Geometry check sheet. Reference: the model listing, model coordinates, mm. A direction names the side the tool comes from. Give positions to 0.01 mm unless a question says otherwise; leave off trailing zeros. Write item = value, one per line. Start each with the question number.
1. Depth check by flat-ended pin: P1, Ø1.3, axis at x = 50.5, z = -3.5, coming from the +Y side; P2, Ø0.6, axis at x = 52.5, z = -1.5, coming from the +Y side; P3, Ø10, axis at y = 2.5, z = 2, coming from the -X side; P4, Ø6, axis at y = 0, z = -9, coming from the +X side. Enter the tip coordinate at first touch or a pass-through.
2. Thickness scan on line 1 along X through (y, z) = (17.35, -4.75); line 2 along X through (y, z) = (8.5, 0); line 3 along Z through (x, y) = (50.5, 17.35) (3 decimals). Record the ranges inside material, lowest first.
3. Mould release check, pull along Y, two halves, no side actions. Record for faces 4 (the cylindrical face through (-52.247, 11.922, 5.734)), 5 (the cylindrical face through (-52.246, 11.984, -10.672)), 6 (the cylindrical face through (51.359, 0.231, 8.797)), 7 (the flat face through (48, 17.25, -5)): pulls with the +Y half, pulls with the -Y half, needs draft (parallel to the pull), parting line crosses it, or undercut.
4. Set-up check for faces 1 (the flat face through (48, 17.25, 0)), 2 (the flat face through (52, 0, -2)), 3 (the cylindrical face through (-52.246, -11.922, -10.734)): record each of +Z, -Z, +X, -X, +Y, -Y from which the full face is reachable in a straight line by a thin tool's end or side.
```python
from build123d import *

# Parameters (mm, degrees)
SKETCH1_W           = 105
SKETCH1_H           = 35
BOSS_EXTRUDE1_DEPTH = 25
CUT_EXTRUDE1_DEPTH  = 0.5
CUT_EXTRUDE2_START  = -0.5
CUT_EXTRUDE2_DEPTH  = 0.5
FILLET1_R           = 4
FILLET2_R           = 1
SKETCH5_R           = 2
CUT_EXTRUDE3_DEPTH  = 0.25
CUT_EXTRUDE4_DEPTH  = 0.25


with BuildPart() as part:
    # Sketch1 → Boss-Extrude1 (new body)
    with BuildSketch(Plane(origin=(0, 0, -15), x_dir=(-1, 0, 0), z_dir=(0, 0, -1))):
        Rectangle(SKETCH1_W, SKETCH1_H)
    extrude(amount=-BOSS_EXTRUDE1_DEPTH)

    # Sketch2 → Cut-Extrude1 (cut)
    with BuildSketch(Plane(origin=(52.5, 0, 0), x_dir=(0, 0, -1), z_dir=(1, 0, 0))):
        with BuildLine():
            Line((-6.875, 9.125), (-6.875, -9.125))
            ThreePointArc((-6.875, -9.125), (-5.703427125, -11.953427125), (-2.875, -13.125))
            Line((-2.875, -13.125), (7.875, -13.125))
            ThreePointArc((7.875, -13.125), (10.703427125, -11.953427125), (11.875, -9.125))
            Line((11.875, -9.125), (11.875, 9.125))
            ThreePointArc((11.875, 9.125), (10.703427125, 11.953427125), (7.875, 13.125))
            Line((7.875, 13.125), (-2.875, 13.125))
            ThreePointArc((-2.875, 13.125), (-5.703427125, 11.953427125), (-6.875, 9.125))
        make_face()
    extrude(amount=-CUT_EXTRUDE1_DEPTH, mode=Mode.SUBTRACT)

    # Sketch3 → Cut-Extrude2 (cut)
    with BuildSketch(Plane.ZY.offset(52.5).offset(CUT_EXTRUDE2_START)):
        with BuildLine():
            Line((2.875, 13.125), (-7.875, 13.125))
            ThreePointArc((-7.875, 13.125), (-10.703427125, 11.953427125), (-11.875, 9.125))
            Line((-11.875, 9.125), (-11.875, -9.125))
            ThreePointArc((-11.875, -9.125), (-10.703427125, -11.953427125), (-7.875, -13.125))
            Line((-7.875, -13.125), (2.875, -13.125))
            ThreePointArc((2.875, -13.125), (5.703427125, -11.953427125), (6.875, -9.125))
            Line((6.875, -9.125), (6.875, 9.125))
            ThreePointArc((6.875, 9.125), (5.703427125, 11.953427125), (2.875, 13.125))
        make_face()
    extrude(amount=CUT_EXTRUDE2_DEPTH, mode=Mode.SUBTRACT)

    # Fillet1
    # the kernel refuses this fillet: 4 mm, written as the material it takes off along each edge
    with BuildSketch(Plane(origin=(-52.5, -27.5, -15), x_dir=(0, 0, 1), z_dir=(0, 1, 0)), Plane(origin=(52.5, 27.5, -15), x_dir=(0, 0, 1), z_dir=(0, -1, 0))) as fillet1_piece_1:
        with BuildLine():
            CenterArc((FILLET1_R, FILLET1_R), FILLET1_R, 180, 90)
            Line((0, FILLET1_R), (0, 0))
            Line((0, 0), (FILLET1_R, 0))
        make_face()
    extrude(amount=55, mode=Mode.SUBTRACT)
    with BuildSketch(Plane(origin=(-52.5, -27.5, 10), x_dir=(0, 0, -1), z_dir=(0, 1, 0)), Plane(origin=(52.5, 27.5, 10), x_dir=(0, 0, -1), z_dir=(0, -1, 0))) as fillet1_piece_2:
        with BuildLine():
            CenterArc((FILLET1_R, -FILLET1_R), FILLET1_R, 90, 90)
            Line((0, -FILLET1_R), (0, 0))
            Line((0, 0), (FILLET1_R, 0))
        make_face()
    extrude(amount=55, mode=Mode.SUBTRACT)

    # Fillet2
    fillet2_edges = [part.edges().sort_by_distance(p)[0] for p in [
        (0, -17.5, -15),
        (0, 17.5, -15),
        (-52.5, 17.5, -2.5),
        (0, 17.5, 10),
        (52.5, 17.5, -2.5),
        (51.328427125, 17.5, 8.828427125),
        (51.328427125, 17.5, -13.828427125),
        (-51.328427125, 17.5, 8.828427125),
        (-51.328427125, 17.5, -13.828427125),
        (-52.5, -17.5, -2.5),
        (52.5, -17.5, -2.5),
        (0, -17.5, 10),
        (51.328427125, -17.5, 8.828427125),
        (51.328427125, -17.5, -13.828427125),
        (-51.328427125, -17.5, 8.828427125),
        (-51.328427125, -17.5, -13.828427125),
    ]]
    fillet(fillet2_edges, radius=FILLET2_R)

    # Sketch5 → Cut-Extrude3 (cut)
    with BuildSketch(Plane(origin=(0, 17.5, 0), x_dir=(1, 0, 0), z_dir=(0, 1, 0))):
        with Locations(Location((47.5, 0.25, 0), (0, 0, 270))):
            Circle(SKETCH5_R)
        with Locations(Location((47.5, 4.75, 0), (0, 0, 270))):
            Circle(SKETCH5_R)
    extrude(amount=-CUT_EXTRUDE3_DEPTH, mode=Mode.SUBTRACT)

    # Sketch6 → Cut-Extrude4 (cut)
    with BuildSketch(Plane(origin=(0, 17.5, 0), x_dir=(1, 0, 0), z_dir=(0, 1, 0))):
        with BuildLine():
            ThreePointArc((50.671391365, 3.65), (50.5, 4.825), (50.328608635, 3.65))
            ThreePointArc((50.328608635, 3.65), (49.9, 3.075), (50.328608635, 2.5))
            ThreePointArc((50.328608635, 2.5), (49.9, 1.925), (50.328608635, 1.35))
            ThreePointArc((50.328608635, 1.35), (50.5, 0.175), (50.671391365, 1.35))
            ThreePointArc((50.671391365, 1.35), (51.1, 1.925), (50.671391365, 2.5))
            ThreePointArc((50.671391365, 2.5), (51.1, 3.075), (50.671391365, 3.65))
        make_face()
    extrude(amount=-CUT_EXTRUDE4_DEPTH, mode=Mode.SUBTRACT)


solid = part.part
```
Answers:
q1.P1 = 17.5
q1.P2 = 17.21
q1.P3 = -52.4
q1.P4 = 52.4
q2.line_1 = -52.03 to 45.5, 49.5 to 50.21, 50.79 to 52.03
q2.line_2 = -52 to 52
q2.line_3 = -13.905 to -4.825, -0.175 to 8.905
q3.face_4 = undercut
q3.face_5 = undercut
q3.face_6 = needs draft
q3.face_7 = pulls with the +Y half
q4.face_1 = +Y
q4.face_2 = +X
q4.face_3 = -X
